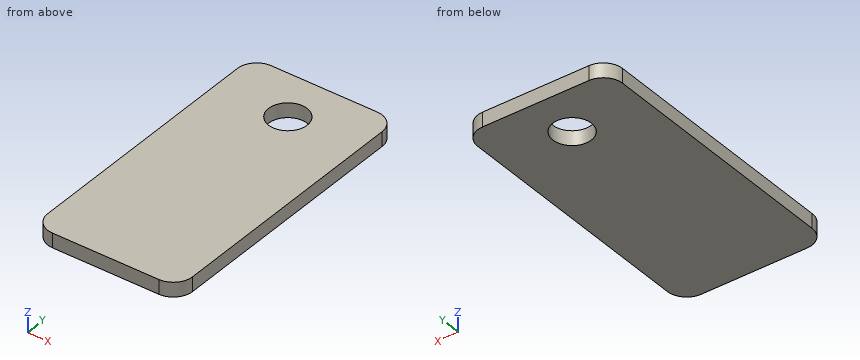
Autodesk Inventor part; units mm, degrees
ref_plane "YZ Plane" through (0, 0, 0) normal (1, 0, 0) x (0, 1, 0)
ref_plane "XZ Plane" through (0, 0, 0) normal (0, 1, 0) x (-1, 0, 0)
ref_plane "XY Plane" through (0, 0, 0) normal (0, 0, 1) x (1, 0, 0)
sketch "Sketch1" plane through (0, 0, 0) normal (0, 0, 1) x (1, 0, 0)
  line L0 (-7.5, 15) -> (7.5, 15)
  line L1 (7.5, 15) -> (7.5, -15)
  line L2 (7.5, -15) -> (-7.5, -15)
  line L3 (-7.5, -15) -> (-7.5, 15)
  circle A0 centre (0, 10) radius 2
  point P0 (0, 0)
  point P1 (-7.5, 0)
  point P2 (0, 15)
  dimension "d0" = 30
  dimension "d1" = 15
  dimension "d5" = 4
  dimension "d7" = 10
extrude "Extrusion1" add sketch "Sketch1" along normal blind 1.5
fillet "Fillet1" radius 2 4 edges at (-7.5, 15, 0.75) (7.5, 15, 0.75) (-7.5, -15, 0.75) (7.5, -15, 0.75)
properties material "Rubber"
Source: CAD feature listing. Evaluate the final solid. Frame: model axes, mm. Coordinates: 2 decimals unless noted, no trailing zeros. Loops run counter-clockwise (first coordinate to the right, second up) from the corner with the lowest first, then second, coordinate; pieces in that order, holes last. Notation, with made-up numbers: (21.25, 82.25) -> (44.25, 82.25) arc R22 cw to (44.25, 121.25) -> close; hole circle Ø7 at (-25, -30). An arc over 180 degrees is marked (long way). One line per item, written item: value. Start each with the question number.
Q1. Section query A-A, the plane x = 0. Return the cut outline in (y, z).
Q2. Contact query for a flat-ended pin moving along its axis: P1, Ø8, axis at x = -5.5, y = -0.5, coming from the -Z side. Output: stop coordinate, or through.
Q3. Line query: line 1 along Y through (x, z) = (0, 0.5); line 2 along X through (y, z) = (10.5, 0.6); line 3 along Y through (x, z) = (-0.5, 0.35). Output: solid intervals per line, ascending.
Q4. Section query C-C, the plane z = 1.05. Return the cut outline in (x, y), and give its area (3 significant figures).
Q5. Section query B-B, the plane y = 10. Return the cut outline in (x, z), and give its area (3 significant figures).
Results:
1. outline: (-15, 0) -> (8, 0) -> (8, 1.5) -> (-15, 1.5) -> close; (12, 0) -> (15, 0) -> (15, 1.5) -> (12, 1.5) -> close
2. P1: z = 0
3. line 1: -15 to 8, 12 to 15
3. line 2: -7.5 to -1.94, 1.94 to 7.5
3. line 3: -15 to 8.06, 11.94 to 15
4. outline: (-7.5, -13) arc R2 ccw to (-5.5, -15) -> (5.5, -15) arc R2 ccw to (7.5, -13) -> (7.5, 13) arc R2 ccw to (5.5, 15) -> (-5.5, 15) arc R2 ccw to (-7.5, 13) -> close; hole circle Ø4 at (0, 10)
4. area: 434 mm^2
5. outline: (-7.5, 0) -> (-2, 0) -> (-2, 1.5) -> (-7.5, 1.5) -> close; (2, 0) -> (7.5, 0) -> (7.5, 1.5) -> (2, 1.5) -> close
5. area: 16.5 mm^2
